Verification items for this drawing (mm, ordinates from the low corner). A direction names the side the tool comes from. Give positions to 0.01 mm unless a question says otherwise; leave off trailing zeros. Order: outer loops, then holes, each group sorted by start corner. A loop starts at its lowest first (then second) coordinate and runs counter-clockwise, first axis right, second up.
(1) Gauge pin test, flat ends, axial feed: pin 1 (3 mm diameter, centred on x = 10.5, y = 3.5, fed in from +Z); pin 2 (2 mm diameter, centred on y = 3.5, z = 6, fed in from +X). Record the tip position at first contact, or that the pin passes through.
(2) Access from +Z, -Z, +X, -X, +Y, -Y to the whole of each face (thin tool, end or side, straight path). Record for the marked faces 4 and 5.
(3) Mould release check, pull along Z, two halves, no side actions. Record for the marked faces 1, 2 and 3: pulls with the +Z half, pulls with the -Z half, needs draft (parallel to the pull), parting line crosses it, or undercut.
(4) Sectioned sample at A-A on x = 6. Record the cut outline in (y, z), plus the area to 3 significant figures.
(5) Scan lines: L1, parallel to Z at x = 2.25, y = 8; L2, parallel to Y at x = 6, z = 5.75; L3, parallel to X at y = 4.5, z = 7.25. Record each from-to range of solid material in increasing order.
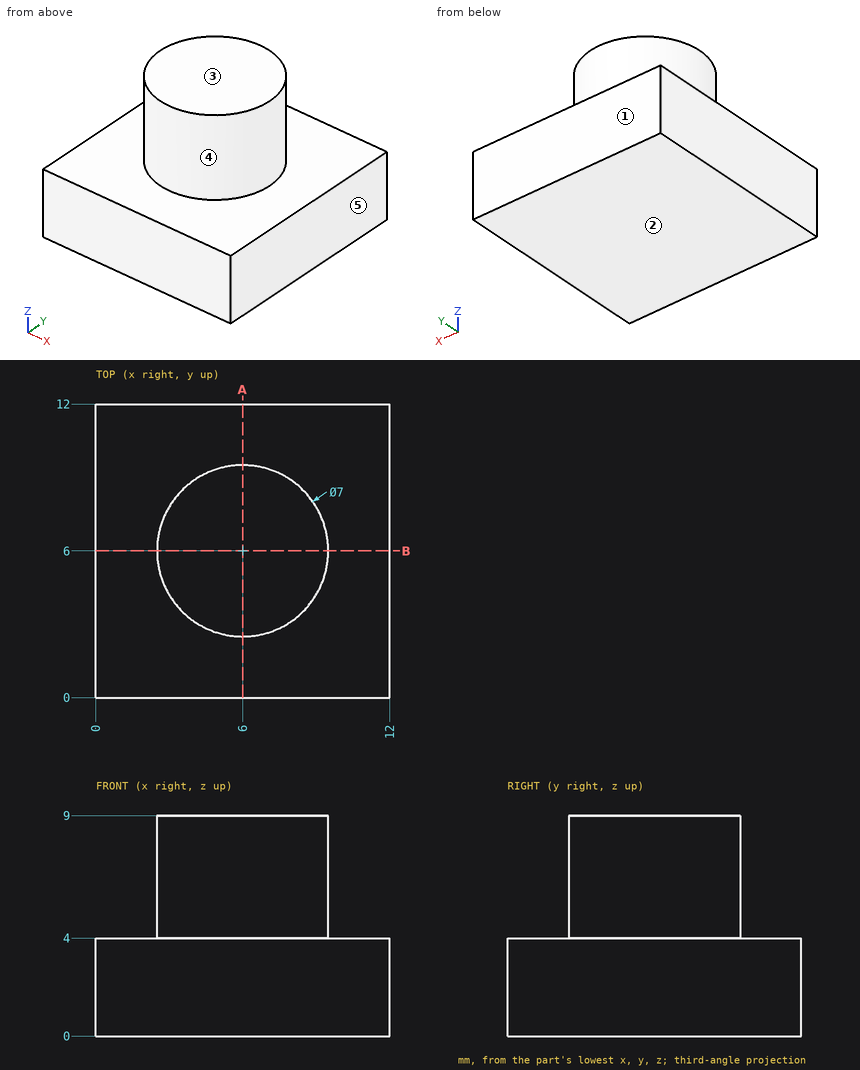
Ans:
1. pin 1: stops at z = 4
1. pin 2: stops at x = 9.16
2. face 4: +Z
2. face 5: +Z, -Z, +X, +Y, -Y
3. face 1: needs draft
3. face 2: pulls with the -Z half
3. face 3: pulls with the +Z half
4. outline: (0, 0) - (12, 0) - (12, 4) - (9.5, 4) - (9.5, 9) - (2.5, 9) - (2.5, 4) - (0, 4) - close
4. area: 83.0 mm2
5. L1: z = 0 to 4
5. L2: y = 2.5 to 9.5
5. L3: x = 2.84 to 9.16
